Input: part model. Units: mm. Frame: model coordinates. Face numbers are marked on the shaded views. A direction names the side the tool comes from. Give positions to 0.01 mm unless a question says otherwise; leave off trailing zeros. Loops run counter-clockwise (first coordinate to the right, second up) from the corner with the lowest first, then second, coordinate; pieces in that order, holes last. Notation, with made-up numbers: M -1.5,40 L 29.5,40 A16 cw 29.5,54 Z; hole C 56.25,-16.5 d2. An arc over 180 degrees is marked long. Answer as a JSON object with one key per item and string values. Group by question number.
1) Section query A-A on y = 3.75. Return loops of the section in (x, z), plus the area to 3 significant figures.
2) Draft query along Z for the marked faces 1, 2 and 3. Return one class per face: +Z half, -Z half, draft (parallel to the pull), parting line (faces both ways), or undercut.
3) Access query for the marked faces 4, 5 and 6. Directions: +Z, -Z, +X, -X, +Y, -Y. A direction counts if a zero-diameter tool reaches every point of the face in a straight line with its end or side. Return the directions, or none.
4) Section query D-D on x = 6. Return loops of the section in (y, z), plus the area to 3 significant figures.
5) Section query B-B on x = 12. Return loops of the section in (y, z).
6) Ray query, L1, parallel to Z at x = 3, y = 0; L2, parallel to Y at x = 10, z = 0; L3, parallel to Y at x = 8.75, z = 0. Return the intervals inside material, ascending.
7) First-contact query: P1, Ø1.3, axis at x = 11, z = -1, coming from the -Y side; P2, Ø1, axis at x = 26.5, z = 11.5, coming from the +Y side; P3, Ø5, axis at x = 30.5, y = 5, coming from the -Z side. Flat tips, straight axial feed; report the tip coordinate or a pass-through.
8) Section query C-C on y = 0. Return loops of the section in (x, z).
from build123d import *

# Parameters (mm, degrees)
SKETCH2_R           = 5
CUT_EXTRUDE1_DEPTH  = 12.5
SKETCH5_R           = 2.95
CUT_EXTRUDE3_DEPTH  = 10
SKETCH14_W          = 15.128379637
SKETCH14_H          = 10
CUT_EXTRUDE4_DEPTH  = 5
SKETCH15_W          = 15.128379637
SKETCH15_H          = 9.028288874
BOSS_EXTRUDE3_DEPTH = 5
FILLET2_R           = 2
FILLET3_R           = 2
CUT_EXTRUDE5_REACH  = 14.15
SKETCH16_R          = 2.25


with BuildPart() as part:
    # Sweep1: sweep along a path in Sketch1
    with BuildLine(Plane(origin=(0, 0, 0), x_dir=(1, 0, 0), z_dir=(0, 1, 0))) as sweep1_path:
        Line((0, 0), (15.128379637, 0))
        ThreePointArc((15.128379637, 0), (19.50794708, -1.010039543), (23.002807262, -3.836122196))
        Line((23.002807262, -3.836122196), (35.409694509, -19.686069062))
    # Sketch2 → Sweep1 (sweep)
    with BuildSketch(Plane(origin=(0, 0, 0), x_dir=(0, 0, -1), z_dir=(1, 0, 0))):
        Circle(SKETCH2_R)
    sweep(path=sweep1_path.line)

    # Sketch4 → Cut-Extrude1 (cut)
    with BuildSketch(Plane.ZY):
        with BuildLine():
            Line((-2.163330765, 2.15), (2.163330765, 2.15))
            ThreePointArc((2.163330765, 2.15), (0, -3.05), (-2.163330765, 2.15))
        make_face()
    extrude(amount=-CUT_EXTRUDE1_DEPTH, mode=Mode.SUBTRACT)

    # Sketch5 → Cut-Extrude3 (cut)
    with BuildSketch(Plane(origin=(23.008372425, 0, 29.393470993), x_dir=(0.787442762, 0, -0.61638778), z_dir=(0.61638778, 0, 0.787442762))):
        with Locations((15.74885525, 0)):
            Circle(SKETCH5_R)
    extrude(amount=-CUT_EXTRUDE3_DEPTH, mode=Mode.SUBTRACT)

    # Sketch14 → Cut-Extrude4 (cut)
    with BuildSketch(Plane.XZ.offset(-2.15)):
        with Locations((7.564189819, 0)):
            Rectangle(SKETCH14_W, SKETCH14_H)
    extrude(amount=-CUT_EXTRUDE4_DEPTH, mode=Mode.SUBTRACT)

    # Sketch15 → Boss-Extrude3 (add)
    with BuildSketch(Plane(origin=(0, 2.15, 0), x_dir=(1, 0, 0), z_dir=(0, 1, 0))):
        with Locations((7.564189819, 0)):
            Rectangle(SKETCH15_W, SKETCH15_H)
    extrude(amount=BOSS_EXTRUDE3_DEPTH)

    # Fillet2
    fillet2_edges = [part.edges().sort_by_distance(p)[0] for p in [
        (7.564189819, 2.15, -4.514144437),
        (7.564189819, 2.15, 4.514144437),
    ]]
    fillet(fillet2_edges, radius=FILLET2_R)

    # Fillet3
    fillet3_edges = [part.edges().sort_by_distance(p)[0] for p in [
        (0, 7.15, 0),
        (7.564189819, 7.15, 4.514144437),
        (15.128379637, 7.15, 0),
        (7.564189819, 7.15, -4.514144437),
    ]]
    fillet(fillet3_edges, radius=FILLET3_R)

    # Sketch16 → Cut-Extrude5 (cut, up to next)
    with BuildSketch(Plane(origin=(0, 7.15, 0), x_dir=(1, 0, 0), z_dir=(0, 1, 0)), mode=Mode.PRIVATE) as cut_extrude5_sk1:
        with Locations((7.564189819, 0)):
            Circle(SKETCH16_R)
    cut_extrude5_tool1 = extrude(cut_extrude5_sk1.sketch, amount=-CUT_EXTRUDE5_REACH, mode=Mode.PRIVATE) & part.part
    add(cut_extrude5_tool1.solids().sort_by_distance((7.56419, 7.15, 0))[0], mode=Mode.SUBTRACT)


solid = part.part
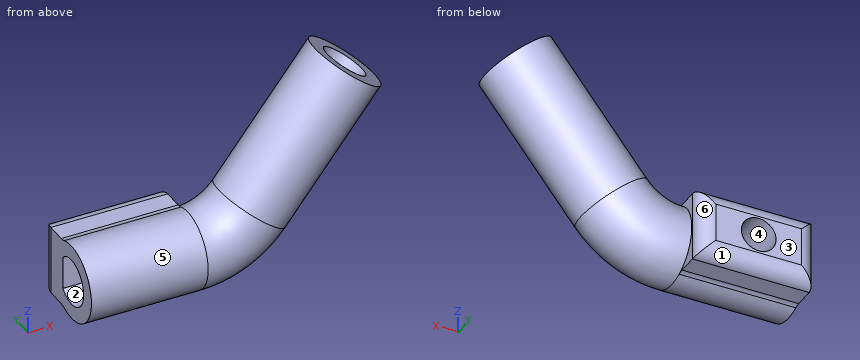
Output:
{
 "1": {"outline": "M 0,-4.51 L 15.13,-4.51 L 15.13,-3.31 A13.31 ccw 25.61,1.8 L 38.01,17.65 L 32.81,21.72 L 20.4,5.87 A6.69 cw 15.13,3.31 L 15.13,4.51 L 0,4.51 Z; hole C 7.56,0 d4.5", "area": "314 mm^2"},
 "2": {"face 1": "-Z half", "face 2": "undercut", "face 3": "draft"},
 "3": {"face 4": "+Y", "face 5": "-X", "face 6": "+Z, -Z, +X, +Y"},
 "4": {"outline": "M 1.83,-4.65 A2 cw 2.56,-4.51 L 5.15,-4.51 A2 ccw 7.15,-2.51 L 7.15,-1.62 L 2.15,-1.62 L 2.15,-2.16 A3.05 cw long 2.15,2.16 L 2.15,1.62 L 7.15,1.62 L 7.15,2.51 A2 ccw 5.15,4.51 L 2.56,4.51 A2 cw 1.83,4.65 A5 ccw long Z", "area": "60.8 mm^2"},
 "5": {"outline": "M 1.83,-4.65 A2 cw 2.56,-4.51 L 5.15,-4.51 A2 ccw 7.15,-2.51 L 7.15,2.51 A2 ccw 5.15,4.51 L 2.56,4.51 A2 cw 1.83,4.65 A5 ccw long Z; hole M 2.15,-2.16 L 2.15,2.16 A3.05 ccw long Z"},
 "6": {"L1": "z = -5 to -3.05, 3.05 to 5", "L2": "y = -5 to -3.05, 2.15 to 7.15", "L3": "y = -5 to -3.05"},
 "7": {"P1": "stops at y = -4.99", "P2": "stops at y = 4.78", "P3": "stops at z = 4.96"},
 "8": {"outline": "M 0,-5 L 15.13,-5 A15 ccw 26.94,0.75 L 39.35,16.6 L 37.73,17.87 L 31.57,9.99 L 26.92,13.63 L 33.09,21.5 L 31.47,22.77 L 19.07,6.92 A5 cw 15.13,5 L 0,5 L 0,3.05 L 12.5,3.05 L 12.5,-3.05 L 0,-3.05 Z"}
}
